Source: CAD feature listing. Evaluate the final solid. Frame: model axes, mm. A direction names the side the tool comes from. Give positions to 0.01 mm unless a question says otherwise; leave off trailing zeros. Loops run counter-clockwise (first coordinate to the right, second up) from the corner with the lowest first, then second, coordinate; pieces in that order, holes last. Notation, with made-up numbers: M 39,48 L 75,48 A25 ccw 75,71 Z; hole C -14.75,42 d4. An arc over 180 degrees is marked long. Answer in a Markdown table with one row per item.
```python
from build123d import *

# Parameters (mm, degrees)
SKETCH1_W           = 120
SKETCH1_H           = 200
BOSS_EXTRUDE1_DEPTH = 3
FILLET1_R           = 60
BOSS_EXTRUDE2_DEPTH = 37.5
FILLET2_R           = 5
SKETCH6_R           = 2.5
CUT_EXTRUDE1_DEPTH  = 37.5
SKETCH7_R           = 5
CUT_EXTRUDE2_DEPTH  = 3
SKETCH9_R           = 8
SKETCH9_R_2         = 2.5
BOSS_EXTRUDE3_DEPTH = 22.5
SKETCH10_R          = 6
CUT_EXTRUDE3_DEPTH  = 3
LPATTERN1_COUNT     = 2
LPATTERN1_PITCH     = 110


with BuildPart() as part:
    # Sketch1 → Boss-Extrude1 (new body)
    with BuildSketch(Plane.XY):
        Rectangle(SKETCH1_W, SKETCH1_H)
    extrude(amount=BOSS_EXTRUDE1_DEPTH)

    # Fillet1
    fillet1_edges = [part.edges().sort_by_distance(p)[0] for p in [
        (60, 100, 1.5),
        (-60, 100, 1.5),
    ]]
    fillet(fillet1_edges, radius=FILLET1_R - 0.0001)  # a hair under: the kernel refuses the full size

    # Sketch4 → Boss-Extrude2 (add)
    with BuildSketch(Plane.XY.offset(3)):
        with BuildLine():
            Line((55, -100), (55, 40))
            ThreePointArc((55, 40), (38.890872965, 78.890872965), (0, 95))
            ThreePointArc((0, 95), (-38.890872965, 78.890872965), (-55, 40))
            Line((-55, 40), (-55, -100))
            Line((-55, -100), (-60, -100))
            Line((-60, -100), (-60, 40))
            ThreePointArc((-60, 40), (-42.426406871, 82.426406871), (0, 100))
            ThreePointArc((0, 100), (42.426406871, 82.426406871), (60, 40))
            Line((60, 40), (60, -100))
            Line((60, -100), (55, -100))
        make_face()
    extrude(amount=BOSS_EXTRUDE2_DEPTH)

    # Fillet2
    fillet2_edges = [part.edges().sort_by_distance(p)[0] for p in [
        (-60, -29.99995, 0),
        (-42.426436161, 82.426436161, 0),
        (-55, -30, 3),
        (0, 95, 3),
        (55, -30, 3),
        (60, -29.99995, 0),
    ]]
    fillet(fillet2_edges, radius=FILLET2_R)

    # Sketch6 → Cut-Extrude1 (cut)
    with BuildSketch(Plane(origin=(60, 0, 0), x_dir=(0, 0, -1), z_dir=(1, 0, 0))):
        with Locations((-33, -75)):
            Circle(SKETCH6_R)
        with Locations((-33, 25)):
            Circle(SKETCH6_R)
    cut_extrude1 = extrude(amount=-CUT_EXTRUDE1_DEPTH, mode=Mode.SUBTRACT)

    # Sketch7 → Cut-Extrude2 (cut)
    with BuildSketch(Plane(origin=(60, 0, 0), x_dir=(0, 0, -1), z_dir=(1, 0, 0))):
        with Locations((-33, 25)):
            Circle(SKETCH7_R)
        with Locations((-33, -75)):
            Circle(SKETCH7_R)
    cut_extrude2 = extrude(amount=-CUT_EXTRUDE2_DEPTH, mode=Mode.SUBTRACT)

    # Mirror1: Cut-Extrude1, Cut-Extrude2 across plane
    add(cut_extrude1.mirror(Plane(origin=(0, 0, 0), x_dir=(0, 0, 1), z_dir=(1, 0, 0))), mode=Mode.SUBTRACT)
    add(cut_extrude2.mirror(Plane(origin=(0, 0, 0), x_dir=(0, 0, 1), z_dir=(1, 0, 0))), mode=Mode.SUBTRACT)

    # Sketch9 → Boss-Extrude3 (add)
    with BuildSketch(Plane.XY.offset(3)):
        with Locations(Location((0, 30, 0), (0, 0, 180))):
            Circle(SKETCH9_R)
        with Locations(Location((0, 30, 0), (0, 0, 180))):
            Circle(SKETCH9_R_2, mode=Mode.SUBTRACT)
    boss_extrude3 = extrude(amount=BOSS_EXTRUDE3_DEPTH)

    # Sketch10 → Cut-Extrude3 (cut)
    with BuildSketch(Plane.XY.offset(3)):
        with Locations((0, 30)):
            Circle(SKETCH10_R)
    cut_extrude3 = extrude(amount=-CUT_EXTRUDE3_DEPTH, mode=Mode.SUBTRACT)

    # LPattern1: Boss-Extrude3, Cut-Extrude3 ×2
    with Locations(*[(0, -i * LPATTERN1_PITCH, 0) for i in range(1, LPATTERN1_COUNT)]):
        add(boss_extrude3)
        add(cut_extrude3, mode=Mode.SUBTRACT)


solid = part.part
```
Q1. Reachability of faces 5 (the flat face through (57, -77, 31)), 6 (the cylindrical face through (1.041, 22.068, 14.092)), 7 (the flat face through (-55, -29, 24)), 8 (the cylindrical face through (-59, 22, 37)), 9 (the cylindrical face through (-0.78, -74.05, 1.52)) from +Z, -Z, +X, -X, +Y, -Y: full face, straight path, thin tool, end or side. Return the list, or none.
Values follow:
| item | result |
|---|---|
| face 5 | +X |
| face 6 | +Z |
| face 7 | +Z, -Y |
| face 8 | -X |
| face 9 | -Z |
Q2. Section query C-C (z = 33). Give the number of separate pieces and of enclosed holes in the cut face, plus the area to 3 significant figures.
Values follow:
| item | result |
|---|---|
| separate pieces | 5 |
| enclosed holes | 0 |
| area | 2,140 mm^2 |
Q3. Ray query, probe 1 along Y at (x, z) = (-55.35, 33); probe 2 along X at (y, z) = (-80, 19); probe 3 along X at (y, z) = (2, 10.5). Return the intervals inside material, ascending. Write a range as from..to.
Values follow:
| item | result |
|---|---|
| probe 1 | -100..-77.5, -72.5..22.5, 27.5..63.16 |
| probe 2 | -60..-55, -8..-2.5, 2.5..8, 55..60 |
| probe 3 | -60..-55, 55..60 |
Q4. Section query B-B (y = -18.5). Output: boundary loops of the cut face in (x, z), plus the area to 3 significant figures.
Values follow:
| item | result |
|---|---|
| outline | M -60,5 A5 ccw -55,0 L 55,0 A5 ccw 60,5 L 60,40.5 L 55,40.5 L 55,8 A5 cw 50,3 L -50,3 A5 cw -55,8 L -55,40.5 L -60,40.5 Z |
| area | 735 mm^2 |
Q5. Section query A-A (z = 12.5). Output: boundary loops of the cut face in (x, y), plus the area to 3 significant figures.
Values follow:
| item | result |
|---|---|
| outline | M -60,-100 L -55,-100 L -55,40 A55 cw 55,40 L 55,-100 L 60,-100 L 60,40 A60 ccw -60,40 Z; C 0,-80 d16; C 0,30 d16; hole C 0,-80 d5; hole C 0,30 d5 |
| area | 2,670 mm^2 |
Q6. Contact query for flat-ended pins moving along their axis: pin 1 Ø8 at (y, z) = (25, 33) entering from +X; pin 2 Ø1.5 at (y, z) = (-28, 4) entering from +X; pin 3 Ø8 at (y, z) = (25, 33) entering from -X. Output: stop coordinate, or through.
Values follow:
| item | result |
|---|---|
| pin 1 | x = 57 |
| pin 2 | x = 59.99 |
| pin 3 | x = -57 |
Q7. Mould query, pull axis Z, two halves, no side actions, for faces 1 (the cylindrical face through (-56.01, -77.22, 31.85)), 2 (the cylindrical face through (58, -31, 1)), 3 (the flat face through (-57, -77, 31)), 4 (the cylindrical face through (-54, -31, 5)). Classes: +Z half, -Z half, draft (parallel to the pull), parting line (faces both ways), or undercut.
Values follow:
| item | result |
|---|---|
| face 1 | undercut |
| face 2 | -Z half |
| face 3 | undercut |
| face 4 | +Z half |
